Check sheet for the modelled part. Datum: model origin and axes. Units: mm. Face numbers are marked on the shaded views. A direction names the side the tool comes from. Round coordinates to 2 decimals unless told otherwise and drop trailing zeros. Order: outer loops, then holes, each group sorted by start corner. A loop starts at its lowest first (then second) coordinate and runs counter-clockwise, first axis right, second up. Notation, with made-up numbers: (-22, 4) -> (6, 4) arc R21 ccw to (6, 10) -> close; hole circle Ø2 at (8, 30.5). An arc over 180 degrees is marked (long way). Use CSV: the item, a comma, the result in double quotes.
Autodesk Inventor part; units mm, degrees
ref_plane "YZ Plane" through (0, 0, 0) normal (1, 0, 0) x (0, 1, 0)
ref_plane "XZ Plane" through (0, 0, 0) normal (0, 1, 0) x (-1, 0, 0)
ref_plane "XY Plane" through (0, 0, 0) normal (0, 0, 1) x (1, 0, 0)
sketch "Boceto2" plane through (0, 0, 0) normal (0, 0, 1) x (1, 0, 0)
  line L0 (0, 0) -> (2000, 0)
  line L1 (2000, 0) -> (2000, 200)
  line L2 (2000, 200) -> (0, 200)
  line L3 (0, 200) -> (0, 0)
  line L4 (0, 0) -> (1000, 0)
  line L5 (1000, 0) -> (1000, 100)
  line L6 (1000, 100) -> (0, 100)
  line L7 (0, 100) -> (0, 0)
  dimension "d0" = 2000
  dimension "d1" = 200
  dimension "d2" = 1000
  dimension "d3" = 100
extrude "Extrusión1" add sketch "Boceto2" along normal blind 400 contours L5 L6 L3 L2 L1 L0
properties part number "3D_Domain"
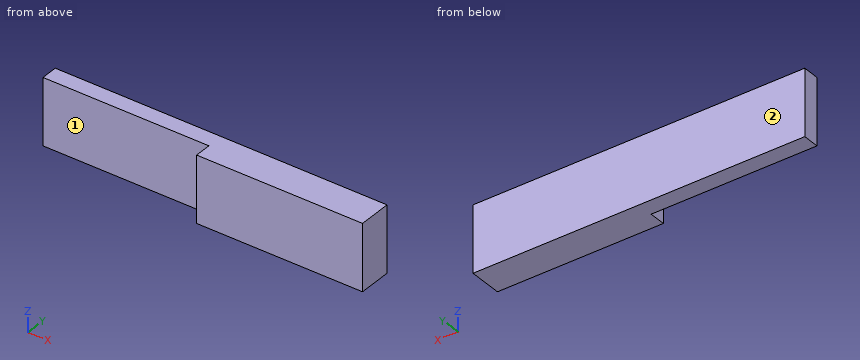
Q1. Go/stop test with a flat-tipped pin: pin 1 (10 mm diameter, centred on y = 82, z = 113, fed in from -X). Record where the tip stops, or that it passes through.
Result sheet:
pin 1,"stops at x = 1000"
Q2. Scan lines: L1, parallel to X at y = 26, z = 289.5; L2, parallel to Y at x = 569, z = 280. Record each from-to range of solid material in increasing order.
Result sheet:
L1,"x = 1000 to 2000"
L2,"y = 100 to 200"
Q3. Sectioned sample at C-C, the plane y = 79. Enter the section's corners in (x, z).
Result sheet:
outline,"(1000, 0) -> (2000, 0) -> (2000, 400) -> (1000, 400) -> close"
Q4. Sectioned sample at B-B, the plane x = 130.5. Enter the section's corners in (y, z), then the cut area to 3 significant figures.
Result sheet:
outline,"(100, 0) -> (200, 0) -> (200, 400) -> (100, 400) -> close"
area,"40,000 mm^2"
Q5. Access from +Z, -Z, +X, -X, +Y, -Y to the whole of each face (thin tool, end or side, straight path). Record for the marked faces 1 and 2.
Result sheet:
face 1,"+Z, -Z, -X, -Y"
face 2,"+Z, -Z, +X, -X, +Y"
Q6. Sectioned sample at A-A, the plane z = 359. Enter the section's corners in (x, y), then the cut area to 3 significant figures.
Result sheet:
outline,"(0, 100) -> (1000, 100) -> (1000, 0) -> (2000, 0) -> (2000, 200) -> (0, 200) -> close"
area,"300,000 mm^2"
